Geometry: final body of the model. Coordinates: model frame, mm. Give positions to 0.01 mm unless a question says otherwise; leave off trailing zeros. Order: outer loops, then holes, each group sorted by start corner. A loop starts at its lowest first (then second) coordinate and runs counter-clockwise, first axis right, second up. Notation, with made-up numbers: (69, 43.25) -> (81, 43.25) arc R27 cw to (81, 80.25) -> close; hole circle Ø11 at (-39.5, 3). An arc over 180 degrees is marked (long way). One line per question, with ' | ' between items.
from build123d import *

# Parameters (mm, degrees)
BOSS_EXTRUDE1_DEPTH = 3.175
CUT_EXTRUDE2_REACH  = 186.942
SKETCH3_W           = 3.175
SKETCH3_H           = 6.35
CUT_EXTRUDE3_REACH  = 186.942
SKETCH4_R           = 2.286
SKETCH5_W           = 6.35
SKETCH5_H           = 3.175
CUT_EXTRUDE4_DEPTH  = 3.175
SKETCH6_W           = 6.35
SKETCH6_H           = 3.175
CUT_EXTRUDE5_DEPTH  = 3.175
SKETCH7_R           = 7.112
SKETCH7_W           = 6.35
SKETCH7_H           = 25.4
CUT_EXTRUDE6_DEPTH  = 3.175


with BuildPart() as part:
    # Sketch1 → Boss-Extrude1 (new body)
    with BuildSketch(Plane(origin=(0, 0, 0), x_dir=(1, 0, 0), z_dir=(0, 1, 0))):
        with BuildLine():
            Line((0, -50.8), (0, 50.8))
            Line((0, 50.8), (127, 50.8))
            ThreePointArc((127, 50.8), (177.8, 0), (127, -50.8))
            Line((127, -50.8), (0, -50.8))
        make_face()
    extrude(amount=BOSS_EXTRUDE1_DEPTH)

    # Sketch3 → Cut-Extrude2 (cut, up to next)
    with BuildSketch(Plane(origin=(0, 3.175, 0), x_dir=(1, 0, 0), z_dir=(0, 1, 0)), mode=Mode.PRIVATE) as cut_extrude2_sk1:
        with Locations((22.5425, 40.64)):
            Rectangle(SKETCH3_W, SKETCH3_H)
    cut_extrude2_tool1 = extrude(cut_extrude2_sk1.sketch, amount=-CUT_EXTRUDE2_REACH, mode=Mode.PRIVATE) & part.part
    # Sketch3 → Cut-Extrude2 (cut, up to next)
    with BuildSketch(Plane(origin=(0, 3.175, 0), x_dir=(1, 0, 0), z_dir=(0, 1, 0)), mode=Mode.PRIVATE) as cut_extrude2_sk2:
        with Locations((66.3575, 40.64)):
            Rectangle(SKETCH3_W, SKETCH3_H)
    cut_extrude2_tool2 = extrude(cut_extrude2_sk2.sketch, amount=-CUT_EXTRUDE2_REACH, mode=Mode.PRIVATE) & part.part
    # Sketch3 → Cut-Extrude2 (cut, up to next)
    with BuildSketch(Plane(origin=(0, 3.175, 0), x_dir=(1, 0, 0), z_dir=(0, 1, 0)), mode=Mode.PRIVATE) as cut_extrude2_sk3:
        with Locations((66.3575, -40.64)):
            Rectangle(SKETCH3_W, SKETCH3_H)
    cut_extrude2_tool3 = extrude(cut_extrude2_sk3.sketch, amount=-CUT_EXTRUDE2_REACH, mode=Mode.PRIVATE) & part.part
    # Sketch3 → Cut-Extrude2 (cut, up to next)
    with BuildSketch(Plane(origin=(0, 3.175, 0), x_dir=(1, 0, 0), z_dir=(0, 1, 0)), mode=Mode.PRIVATE) as cut_extrude2_sk4:
        with Locations((22.5425, -40.64)):
            Rectangle(SKETCH3_W, SKETCH3_H)
    cut_extrude2_tool4 = extrude(cut_extrude2_sk4.sketch, amount=-CUT_EXTRUDE2_REACH, mode=Mode.PRIVATE) & part.part
    add(cut_extrude2_tool1.solids().sort_by_distance((22.5425, 3.175, -40.64))[0], mode=Mode.SUBTRACT)
    add(cut_extrude2_tool2.solids().sort_by_distance((66.3575, 3.175, -40.64))[0], mode=Mode.SUBTRACT)
    add(cut_extrude2_tool3.solids().sort_by_distance((66.3575, 3.175, 40.64))[0], mode=Mode.SUBTRACT)
    add(cut_extrude2_tool4.solids().sort_by_distance((22.5425, 3.175, 40.64))[0], mode=Mode.SUBTRACT)

    # Sketch4 → Cut-Extrude3 (cut, up to next)
    with BuildSketch(Plane(origin=(0, 3.175, 0), x_dir=(1, 0, 0), z_dir=(0, 1, 0)), mode=Mode.PRIVATE) as cut_extrude3_sk1:
        with Locations(Location((139.7, 25.4, 0), (0, 0, 270))):
            Circle(SKETCH4_R)
    cut_extrude3_tool1 = extrude(cut_extrude3_sk1.sketch, amount=-CUT_EXTRUDE3_REACH, mode=Mode.PRIVATE) & part.part
    # Sketch4 → Cut-Extrude3 (cut, up to next)
    with BuildSketch(Plane(origin=(0, 3.175, 0), x_dir=(1, 0, 0), z_dir=(0, 1, 0)), mode=Mode.PRIVATE) as cut_extrude3_sk2:
        with Locations(Location((139.7, -25.4, 0), (0, 0, 90))):
            Circle(SKETCH4_R)
    cut_extrude3_tool2 = extrude(cut_extrude3_sk2.sketch, amount=-CUT_EXTRUDE3_REACH, mode=Mode.PRIVATE) & part.part
    add(cut_extrude3_tool1.solids().sort_by_distance((139.7, 3.175, -25.4))[0], mode=Mode.SUBTRACT)
    add(cut_extrude3_tool2.solids().sort_by_distance((139.7, 3.175, 25.4))[0], mode=Mode.SUBTRACT)

    # Sketch5 → Cut-Extrude4 (cut)
    with BuildSketch(Plane(origin=(0, 3.175, 0), x_dir=(1, 0, 0), z_dir=(0, 1, 0))):
        with Locations((139.7, -12.7)):
            Rectangle(SKETCH5_W, SKETCH5_H)
        with Locations((139.7, 12.7)):
            Rectangle(SKETCH5_W, SKETCH5_H)
    extrude(amount=-CUT_EXTRUDE4_DEPTH, mode=Mode.SUBTRACT)

    # Sketch6 → Cut-Extrude5 (cut)
    with BuildSketch(Plane(origin=(0, 3.175, 0), x_dir=(1, 0, 0), z_dir=(0, 1, 0))):
        with Locations((44.45, 40.64)):
            Rectangle(SKETCH6_W, SKETCH6_H)
        with Locations((44.45, -40.64)):
            Rectangle(SKETCH6_W, SKETCH6_H)
        with Locations((57.15, 40.64)):
            Rectangle(SKETCH6_W, SKETCH6_H)
        with Locations((31.75, 40.64)):
            Rectangle(SKETCH6_W, SKETCH6_H)
        with Locations((31.75, -40.64)):
            Rectangle(SKETCH6_W, SKETCH6_H)
        with Locations((57.15, -40.64)):
            Rectangle(SKETCH6_W, SKETCH6_H)
    extrude(amount=-CUT_EXTRUDE5_DEPTH, mode=Mode.SUBTRACT)

    # Sketch7 → Cut-Extrude6 (cut)
    with BuildSketch(Plane(origin=(0, 3.175, 0), x_dir=(1, 0, 0), z_dir=(0, 1, 0))):
        with Locations(Location((101.6, 0, 0), (0, 0, 270))):
            Circle(SKETCH7_R)
        with Locations((76.2, 0)):
            Rectangle(SKETCH7_W, SKETCH7_H)
    extrude(amount=-CUT_EXTRUDE6_DEPTH, mode=Mode.SUBTRACT)


solid = part.part
1) Pull-direction query (Z, two-part tool) for faces 1 (the flat face through (20.955, 2, 41)), 2 (the cylindrical face through (177.788, 1.565, -1.117)), 3 (the flat face through (0, 2, 1)); classes: +Z half, -Z half, draft (parallel to the pull), parting line (faces both ways), or undercut.
Check result:
face 1: undercut | face 2: parting line | face 3: draft
2) Material intervals for probe 1 along Z at (x, y) = (139.7, 0.75); probe 2 along Z at (x, y) = (23, 0.45) (3 decimals); probe 3 along X at (y, z) = (2.95, -14) (3 decimals), sorted ascending. Write a range as from..to.
Check result:
probe 1: z = -49.19..-27.69, -23.11..-14.29, -11.11..11.11, 14.29..23.11, 27.69..49.19 | probe 2: z = -50.8..-43.815, -37.465..37.465, 43.815..50.8 | probe 3: x = 0..136.525, 142.875..175.833
3) Section C-C on x = 139.7. Return loops of the section in (y, z) (1 decimal).
Check result:
outline: (0, -49.2) -> (3.2, -49.2) -> (3.2, -27.7) -> (0, -27.7) -> close; (0, -23.1) -> (3.2, -23.1) -> (3.2, -14.3) -> (0, -14.3) -> close; (0, -11.1) -> (3.2, -11.1) -> (3.2, 11.1) -> (0, 11.1) -> close; (0, 14.3) -> (3.2, 14.3) -> (3.2, 23.1) -> (0, 23.1) -> close; (0, 27.7) -> (3.2, 27.7) -> (3.2, 49.2) -> (0, 49.2) -> close
4) Contact query for flat-ended pins moving along their axis: pin 1 Ø1.5 at (y, z) = (0.5, -37.5) entering from -X; pin 2 Ø1.6 at (y, z) = (1, 39.5) entering from +X. Output: stop coordinate, or through.
Check result:
pin 1: stops at x = 0 | pin 2: stops at x = 159.91
5) Section B-B on z = 0. Return loops of the section in (x, y) (3 decimals), plus the area to 3 significant figures.
Check result:
outline: (0, 0) -> (73.025, 0) -> (73.025, 3.175) -> (0, 3.175) -> close; (79.375, 0) -> (94.488, 0) -> (94.488, 3.175) -> (79.375, 3.175) -> close; (108.712, 0) -> (177.8, 0) -> (177.8, 3.175) -> (108.712, 3.175) -> close | area: 499 mm^2
6) Section D-D on z = -25.4. Return loops of the section in (x, y) (3 decimals).
Check result:
outline: (0, 0) -> (137.414, 0) -> (137.414, 3.175) -> (0, 3.175) -> close; (141.986, 0) -> (170.994, 0) -> (170.994, 3.175) -> (141.986, 3.175) -> close
7) Section A-A on x = 101.6. Return loops of the section in (y, z) (3 decimals), plus the area to 3 significant figures.
Check result:
outline: (0, -50.8) -> (3.175, -50.8) -> (3.175, -7.112) -> (0, -7.112) -> close; (0, 7.112) -> (3.175, 7.112) -> (3.175, 50.8) -> (0, 50.8) -> close | area: 277 mm^2
